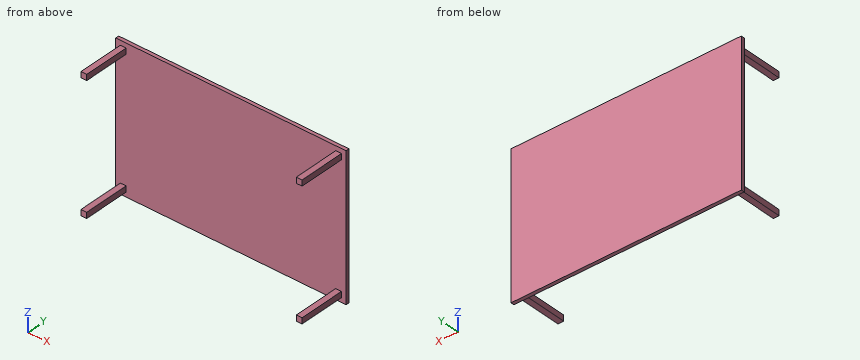
from build123d import *

# Parameters (mm, degrees)
SKETCH1_W             = 25
SKETCH1_H             = 25
BOSS_EXTRUDE1_DEPTH   = 200
BOSS_EXTRUDE1_2_DEPTH = 200
BOSS_EXTRUDE1_3_DEPTH = 200
BOSS_EXTRUDE1_4_DEPTH = 200
SKETCH2_W             = 1000
SKETCH2_H             = 620
BOSS_EXTRUDE2_DEPTH   = 15


with BuildPart() as part:
    # Sketch1 → Boss-Extrude1 (new body)
    with BuildSketch(Plane(origin=(0, 0, 0), x_dir=(1, 0, 0), z_dir=(0, 1, 0))):
        with Locations((-467.5, -277.5)):
            Rectangle(SKETCH1_W, SKETCH1_H)
    extrude(amount=BOSS_EXTRUDE1_DEPTH)



with BuildPart() as body_2:
    # Sketch1 → Boss-Extrude1 2 (new body)
    with BuildSketch(Plane(origin=(0, 0, 0), x_dir=(1, 0, 0), z_dir=(0, 1, 0))):
        with Locations((-467.5, 277.5)):
            Rectangle(SKETCH1_W, SKETCH1_H)
    extrude(amount=BOSS_EXTRUDE1_2_DEPTH)


with BuildPart() as body_3:
    # Sketch1 → Boss-Extrude1 3 (new body)
    with BuildSketch(Plane(origin=(0, 0, 0), x_dir=(1, 0, 0), z_dir=(0, 1, 0))):
        with Locations((467.5, 277.5)):
            Rectangle(SKETCH1_W, SKETCH1_H)
    extrude(amount=BOSS_EXTRUDE1_3_DEPTH)


with BuildPart() as body_4:
    # Sketch1 → Boss-Extrude1 4 (new body)
    with BuildSketch(Plane(origin=(0, 0, 0), x_dir=(1, 0, 0), z_dir=(0, 1, 0))):
        with Locations((467.5, -277.5)):
            Rectangle(SKETCH1_W, SKETCH1_H)
    extrude(amount=BOSS_EXTRUDE1_4_DEPTH)


with BuildPart() as part_1:
    add(part.part)

    add(body_2.part)  # Boss-Extrude2 merges body 2

    add(body_3.part)  # Boss-Extrude2 merges body 3

    add(body_4.part)  # Boss-Extrude2 merges body 4
    # Sketch2 → Boss-Extrude2 (add)
    with BuildSketch(Plane(origin=(0, 200, 0), x_dir=(1, 0, 0), z_dir=(0, 1, 0))):
        Rectangle(SKETCH2_W, SKETCH2_H)
    extrude(amount=BOSS_EXTRUDE2_DEPTH)


solid = part_1.part
Geometry: final body of the model. Coordinates: model frame, mm. Coordinates: 2 decimals unless noted, no trailing zeros. Loops run counter-clockwise (first coordinate to the right, second up) from the corner with the lowest first, then second, coordinate; pieces in that order, holes last. Notation, with made-up numbers: (33.25, 71.25) - (63.25, 71.25) arc R20 cw to (63.25, 89.25) - close; hole circle Ø5 at (-28.75, -37). An arc over 180 degrees is marked (long way). Put each result on its own line as item: value. Start each with the question number.
Q1. Line query: line 1 (X direction, y = 113, z = 266); line 2 (Y direction, x = -163, z = -97). Output: solid intervals per line, ascending.
Q2. Cut plane A-A, the plane y = 37. Return loops of the section in (x, z), and give its area (3 significant figures).
Q3. Cut plane B-B, the plane x = 425.5. Return loops of the section in (y, z), and give its area (3 significant figures).
Q4. Pin query (flat end, axial travel): pin 1 Ø7.5 at (x, y) = (472.5, 133.5) entering from +Z; pin 2 Ø12.5 at (x, y) = (465.5, 72.5) entering from -Z; pin 3 Ø3 at (x, z) = (-56.5, 215.5) entering from -Y. Return the tip coordinate at first contact, or that it passes through.
Q5. Cut plane C-C, the plane z = 189. Return loops of the section in (x, y).
Filled sheet:
1. line 1: -480 to -455, 455 to 480
1. line 2: 200 to 215
2. outline: (-480, -290) - (-455, -290) - (-455, -265) - (-480, -265) - close; (-480, 265) - (-455, 265) - (-455, 290) - (-480, 290) - close; (455, -290) - (480, -290) - (480, -265) - (455, -265) - close; (455, 265) - (480, 265) - (480, 290) - (455, 290) - close
2. area: 2,500 mm²
3. outline: (200, -310) - (215, -310) - (215, 310) - (200, 310) - close
3. area: 9,300 mm²
4. pin 1: z = 290
4. pin 2: z = -290
4. pin 3: y = 200
5. outline: (-500, 200) - (500, 200) - (500, 215) - (-500, 215) - close
